Design review of the part built by this model. Coordinates are the model's own, in mm. Give positions to 0.01 mm unless a question says otherwise; leave off trailing zeros. Write each loop counter-clockwise with the first axis right and the second up, starting at its lowest first coordinate (ties: lowest second). Pieces come first, ordered by that corner, then holes.
```python
from build123d import *

# Parameters (mm, degrees)
PAD_DEPTH  = 50.8
SKETCH_R   = 4.4
HOLE_DEPTH = 50.801


with BuildPart() as part:
    # Sketch001 → Pad (new body)
    with BuildSketch(Plane.XY):
        with BuildLine():
            ThreePointArc((0, 88.9991), (-58.64132, 31.921047), (-74.045407, -48.449486))
            ThreePointArc((-74.045407, -48.449486), (-2.377196, -69.495491), (70.107976, -51.46311))
            ThreePointArc((70.107976, -51.46311), (57.587958, 30.015227), (0, 88.9991))
        make_face()
    extrude(amount=PAD_DEPTH)

    # Sketch (on Sketch) → Hole (cut, through all)
    with BuildSketch(Plane(origin=(0, 0, 0), x_dir=(-1, 0, 0), z_dir=(0, 0, -1))):
        with Locations((-60.575023, -34.979102)):
            Circle(SKETCH_R)
        with Locations((0, 69.9491)):
            Circle(SKETCH_R)
        with Locations((60.582976, -34.965326)):
            Circle(SKETCH_R)
    extrude(amount=-HOLE_DEPTH, mode=Mode.SUBTRACT)


solid = part.part
```
(1) To check wall thickness, follow L1, parallel to Y at x = 0, z = 21; L2, parallel to X at y = -34, z = 22; L3, parallel to Y at x = 59, z = 11.5. State the ranges of each line that lie inside material, in increasing order.
Resolved:
L1: y = -69.53 to 65.55, 74.35 to 89
L2: x = -74.95 to -64.88, -56.29 to 56.29, 64.86 to 71.74
L3: y = -57.04 to -39.09, -30.87 to 27.1
(2) Consider section A-A, the plane x = 58. Give the boundary of the cut face in (y, z).
Resolved:
outline: (-57.48, 0) - (-38.55, 0) - (-38.55, 50.8) - (-57.48, 50.8) - close; (-31.41, 0) - (29.18, 0) - (29.18, 50.8) - (-31.41, 50.8) - close
(3) Mouldability with a two-part tool opening along X and no side actions: class faces 1 (the face through (0.954, 65.654, 25.044)), 2 (the face through (-3, -7, 50.8)), 3 (the face through (-58.085, 32.943, 25.044)) as pulls with the +X half, pulls with the -X half, needs draft (parallel to the pull), parting line crosses it, or undercut.
Resolved:
face 1: undercut
face 2: needs draft
face 3: pulls with the -X half
(4) Consider section D-D, the plane y = 0. Give the boundary of the cut face in (x, z).
Resolved:
outline: (-70.96, 0) - (68.36, 0) - (68.36, 50.8) - (-70.96, 50.8) - close
(5) Consider section B-B, the plane y = -37. Give the boundary of the cut face in (x, z), then the cut area to 3 significant figures.
Resolved:
outline: (-74.89, 0) - (-64.48, 0) - (-64.48, 50.8) - (-74.89, 50.8) - close; (-56.68, 0) - (56.67, 0) - (56.67, 50.8) - (-56.68, 50.8) - close; (64.48, 0) - (71.62, 0) - (71.62, 50.8) - (64.48, 50.8) - close
area: 6,650 mm2
(6) Clearance check with flat-ended pins moving along their axes: P1, Ø2, axis at y = -14, z = 32, coming from the -X side; P2, Ø6, axis at y = 46, z = 44, coming from the +X side; P3, Ø1.5, axis at x = 41.5, z = 14.5, coming from the -Y side. State where each tip first meets the part, or that it passes through.
Resolved:
P1: stops at x = -73.79
P2: stops at x = 50.18
P3: stops at y = -63.77
(7) Consider section C-C, the plane z = 30. Give the boundary of the cut face in (x, y).
Resolved:
outline: (-74.05, -48.45) arc R142.74 ccw to (70.11, -51.46) arc R134.91 ccw to (0, 89) arc R136.36 ccw to start; hole circle Ø8.8 at (-60.58, -34.97); hole circle Ø8.8 at (0, 69.95); hole circle Ø8.8 at (60.58, -34.98)
